Geometry: final body of the model. Coordinates: model frame, mm. Give positions to 0.01 mm unless a question says otherwise; leave off trailing zeros. Loops run counter-clockwise (first coordinate to the right, second up) from the corner with the lowest first, then second, coordinate; pieces in that order, holes last.
```python
from build123d import *

# Parameters (mm, degrees)
SKETCH_2_R               = 37.5
SKETCH_2_R_2             = 34.5
EXTRUDE_1_DEPTH          = 59.5
CUT_EXTRUDE_1_REACH      = 81.704
CUT_EXTRUDE_1_END_RADIUS = 37.5
CUT_EXTRUDE_2_REACH      = 81.704
CUT_EXTRUDE_2_END_RADIUS = 37.5
SKETCH_4_W               = 119
SKETCH_4_H               = 2


with BuildPart() as part:
    # 草图2 → 凸台-拉伸1 (new, symmetric)
    with BuildSketch(Plane.XY):
        Circle(SKETCH_2_R)
        Circle(SKETCH_2_R_2, mode=Mode.SUBTRACT)
    extrude(amount=EXTRUDE_1_DEPTH, both=True)

    # 切除-拉伸1: up to this cylinder (the profile starts inside it)
    cut_extrude_1_end = Plane(origin=(0, 0, -50.003604), z_dir=(0, 0, -1)) * Cylinder(CUT_EXTRUDE_1_END_RADIUS, 239.408, mode=Mode.PRIVATE)
    # 草图3 → 切除-拉伸1 (cut, up to the surface)
    with BuildSketch(Plane(origin=(0, 0, 0), x_dir=(0, 0, -1), z_dir=(1, 0, 0)), mode=Mode.PRIVATE) as cut_extrude_1_sk1:
        with BuildLine():
            Line((44.5, -5), (59.5, -5))
            Line((59.5, -5), (59.5, 5))
            Line((59.5, 5), (44.5, 5))
            ThreePointArc((44.5, 5), (39.5, 0), (44.5, -5))
        make_face()
    cut_extrude_1_tool1 = extrude(cut_extrude_1_sk1.sketch, amount=-CUT_EXTRUDE_1_REACH, mode=Mode.PRIVATE) & cut_extrude_1_end
    add(cut_extrude_1_tool1.solids().sort_by_distance((0, 0, -50.003604))[0], mode=Mode.SUBTRACT)

    # 切除-拉伸2: up to this cylinder (the profile starts inside it)
    cut_extrude_2_end = Plane(origin=(0, 0, 0), z_dir=(0, 0, -1)) * Cylinder(CUT_EXTRUDE_2_END_RADIUS, 239.408, mode=Mode.PRIVATE)
    # 草图4 → 切除-拉伸2 (cut, up to the surface)
    with BuildSketch(Plane(origin=(0, 0, 0), x_dir=(0, 0, -1), z_dir=(1, 0, 0)), mode=Mode.PRIVATE) as cut_extrude_2_sk1:
        Rectangle(SKETCH_4_W, SKETCH_4_H)
    cut_extrude_2_tool1 = extrude(cut_extrude_2_sk1.sketch, amount=-CUT_EXTRUDE_2_REACH, mode=Mode.PRIVATE) & cut_extrude_2_end
    add(cut_extrude_2_tool1.solids().sort_by_distance((0, 0, 0))[0], mode=Mode.SUBTRACT)


solid = part.part
```
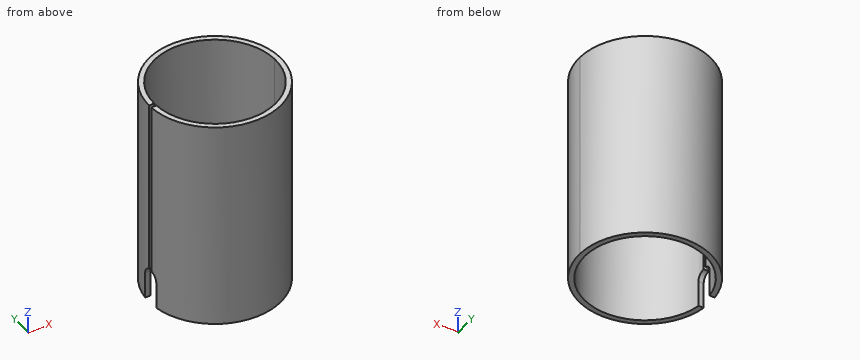
Q1. Material intervals for probe 1 along Y at (x, z) = (1, -25); probe 2 along Y at (x, z) = (16.5, -25); probe 3 along X at (y, z) = (-14.5, 6), sorted ascending.
Q2. Section query B-B, the plane x = -26. Return loops of the section in (y, z).
Q3. Section query A-A, the plane y = -24.5. Return loops of the section in (x, z), and give its area (3 significant figures).
Q4. Pin query (flat end, axial travel): pin 1 Ø10 at (y, z) = (10, -41) entering from -X; pin 2 Ø2.5 at (x, z) = (-36, -54) entering from +Y; pin 3 Ø1.5 at (x, z) = (-35.5, -55) entering from -Y; pin 4 Ø2 at (x, y) = (-28, -27.5) entering from +Z. Return the tip coordinate at first contact, or that it passes through.
Q5. Section query C-C, the plane z = -19.5. Return loops of the section in (x, y).
Resolved:
1. probe 1: y = -37.49 to -34.49, 34.49 to 37.49
1. probe 2: y = -33.67 to -30.3, 30.3 to 33.67
1. probe 3: x = -34.58 to -31.3, 31.3 to 34.58
2. outline: (-27.02, -59.5) - (-22.68, -59.5) - (-22.68, 59.5) - (-27.02, 59.5) - close; (22.68, -59.5) - (27.02, -59.5) - (27.02, 59.5) - (22.68, 59.5) - close
3. outline: (-28.39, -59.5) - (-24.29, -59.5) - (-24.29, 59.5) - (-28.39, 59.5) - close; (24.29, -59.5) - (28.39, -59.5) - (28.39, 59.5) - (24.29, 59.5) - close
3. area: 976 mm2
4. pin 1: stops at x = -37.17
4. pin 2: stops at y = 14.1
4. pin 3: stops at y = -14.1
4. pin 4: passes through
5. outline: (-37.49, -1) arc R37.5 ccw (long way) to (-37.49, 1) - (-34.49, 1) arc R34.5 cw (long way) to (-34.49, -1) - close
